Input: part model. Units: mm. Frame: model coordinates. Give positions to 0.01 mm unless a question says otherwise; leave off trailing zeros. Loops run counter-clockwise (first coordinate to the right, second up) from the corner with the lowest first, then second, coordinate; pieces in that order, holes last.
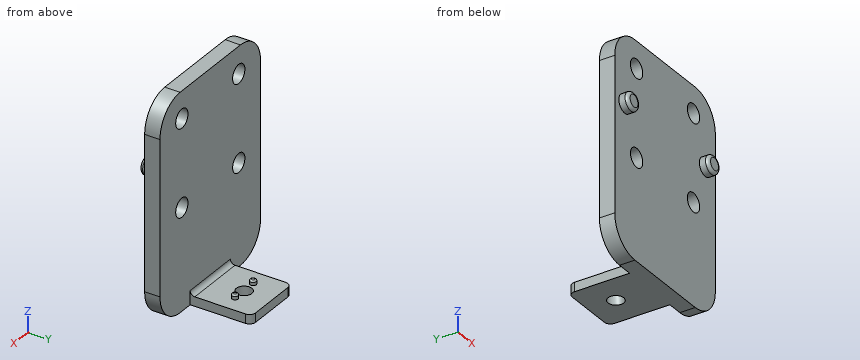
from build123d import *

# Parameters (mm, degrees)
SKETCH_1_W          = 50
SKETCH_1_H          = 70
EXTRUDE_1_DEPTH     = 5
SKETCH_2_R          = 3.05
CUT_EXTRUDE_1_DEPTH = 54.53308254
SKETCH_4_R          = 2.95
EXTRUDE_2_DEPTH     = 3
FILLET_1_R          = 1
FILLET_2_R          = 10
SKETCH_6_W          = 20
SKETCH_6_H          = 3
EXTRUDE_3_DEPTH     = 20
EXTRUDE_5_DEPTH     = 20
FILLET_3_R          = 2
SKETCH_9_R          = 2.55
CUT_EXTRUDE_2_DEPTH = 76.756187866
EXTRUDE_START       = 1.5
SKETCH_9_4_R        = 1
SKETCH_9_4_R_2      = 2.55
EXTRUDE_6_DEPTH     = 1.5
FILLET_4_R          = 0.5


with BuildPart() as part:
    # Sketch 1 → Extrude 1 (new body)
    with BuildSketch(Plane(origin=(0, 0, 0), x_dir=(1, 0, 0), z_dir=(0, 1, 0))):
        with Locations((0, 12.072188459)):
            Rectangle(SKETCH_1_W, SKETCH_1_H)
    extrude(amount=EXTRUDE_1_DEPTH)

    # Sketch 2 → Cut-Extrude 1 (cut, through all)
    with BuildSketch(Plane(origin=(0, 5, 0), x_dir=(1, 0, 0), z_dir=(0, 1, 0))):
        with Locations(Location((14.142135624, 14.142135624, 0), (0, 0, 270))):
            Circle(SKETCH_2_R)
        with Locations(Location((14.142135624, -14.142135624, 0), (0, 0, 270))):
            Circle(SKETCH_2_R)
        with Locations(Location((-14.142135624, -14.142135624, 0), (0, 0, 270))):
            Circle(SKETCH_2_R)
        with Locations(Location((-14.142135624, 14.142135624, 0), (0, 0, 270))):
            Circle(SKETCH_2_R)
    extrude(amount=-CUT_EXTRUDE_1_DEPTH, mode=Mode.SUBTRACT)

    # Sketch 4 → Extrude 2 (add)
    with BuildSketch(Plane.XZ):
        with Locations(Location((20, 0, 0), (0, 0, 90))):
            Circle(SKETCH_4_R)
        with Locations(Location((-20, 0, 0), (0, 0, 90))):
            Circle(SKETCH_4_R)
    extrude(amount=EXTRUDE_2_DEPTH)

    # Fillet 1
    fillet_1_edges = [part.edges().sort_by_distance(p)[0] for p in [
        (20, -3, -2.95),
        (-20, -3, -2.95),
    ]]
    fillet(fillet_1_edges, radius=FILLET_1_R)

    # Fillet 2
    fillet_2_edges = [part.edges().sort_by_distance(p)[0] for p in [
        (-25, 2.5, -47.072188459),
        (25, 2.5, -47.072188459),
        (25, 2.5, 22.927811541),
        (-25, 2.5, 22.927811541),
    ]]
    fillet(fillet_2_edges, radius=FILLET_2_R)

    # Sketch 6 → Extrude 3 (add)
    with BuildSketch(Plane(origin=(0, 5, 0), x_dir=(1, 0, 0), z_dir=(0, 1, 0))):
        with Locations((0, 45.572188459)):
            Rectangle(SKETCH_6_W, SKETCH_6_H)
    extrude(amount=EXTRUDE_3_DEPTH)

    # Sketch 8 → Extrude 5 (add)
    with BuildSketch(Plane.ZY.offset(10)):
        with BuildLine():
            Line((-44.072188459, 6.5), (-44.072188459, 5))
            Line((-44.072188459, 5), (-42.572188459, 5))
            ThreePointArc((-42.572188459, 5), (-43.63284863, 5.439339828), (-44.072188459, 6.5))
        make_face()
    extrude(amount=-EXTRUDE_5_DEPTH)

    # Fillet 3
    fillet_3_edges = [part.edges().sort_by_distance(p)[0] for p in [
        (-10, 25, -45.572188459),
        (10, 25, -45.572188459),
    ]]
    fillet(fillet_3_edges, radius=FILLET_3_R)

    # Sketch 9 → Cut-Extrude 2 (cut, through all)
    with BuildSketch(Plane.XY.offset(-44.072188459)):
        with Locations((0, 16)):
            Circle(SKETCH_9_R)
    extrude(amount=-CUT_EXTRUDE_2_DEPTH, mode=Mode.SUBTRACT)

    # Sketch 9_4 → Extrude 6 (add)
    with BuildSketch(Plane.XY.offset(-44.072188459).offset(EXTRUDE_START)):
        with Locations(Location((-4.5, 16, 0), (0, 0, 180))):
            Circle(SKETCH_9_4_R)
        with Locations(Location((4.5, 16, 0), (0, 0, 180))):
            Circle(SKETCH_9_4_R)
        with Locations((0, 16)):
            Circle(SKETCH_9_4_R_2)
    extrude(amount=-EXTRUDE_6_DEPTH)


with BuildPart() as extrude_6_kept_piece:
    # of the separate pieces the step leaves, the one the design keeps (extrude_6_pieces_kept)
    add(part.part.solids().sort_by_distance((10, 23, -47.072188459))[0])

    # Fillet 4
    fillet_4_edges = [extrude_6_kept_piece.edges().sort_by_distance(p)[0] for p in [
        (-3.5, 16, -42.572188459),
        (5.5, 16, -42.572188459),
    ]]
    fillet(fillet_4_edges, radius=FILLET_4_R)


solid = extrude_6_kept_piece.part
(1) Cut plane A-A (z = -15). Return the cut outline in (x, y), and give its area (3 significant figures).
Values follow:
outline: (-25, 0) - (-17.07, 0) - (-17.07, 5) - (-25, 5) - close; (-11.22, 0) - (11.22, 0) - (11.22, 5) - (-11.22, 5) - close; (17.07, 0) - (25, 0) - (25, 5) - (17.07, 5) - close
area: 191 mm2
(2) Cut plane C-C (y = 2.5). Return the cut outline in (x, z).
Values follow:
outline: (-25, -37.07) arc R10 ccw to (-15, -47.07) - (15, -47.07) arc R10 ccw to (25, -37.07) - (25, 12.93) arc R10 ccw to (15, 22.93) - (-15, 22.93) arc R10 ccw to (-25, 12.93) - close; hole circle Ø6.1 at (-14.14, -14.14); hole circle Ø6.1 at (-14.14, 14.14); hole circle Ø6.1 at (14.14, -14.14); hole circle Ø6.1 at (14.14, 14.14)
(3) Pin query (flat end, axial travel): pin 1 Ø0.5 at (x, y) = (-4.5, 16) entering from +Z; pin 2 Ø5 at (y, z) = (14.5, -44.5) entering from -X; pin 3 Ø8 at (y, z) = (15.5, -39) entering from +X. Return the tip coordinate at first contact, or that it passes through.
Values follow:
pin 1: stops at z = -42.57
pin 2: stops at x = -10
pin 3: stops at x = 5.49
(4) Cut plane B-B (x = -16). Return the cut outline in (y, z), and give its area (3 significant figures).
Values follow:
outline: (0, -47.02) - (5, -47.02) - (5, -16.56) - (0, -16.56) - close; (0, -11.72) - (5, -11.72) - (5, 11.72) - (0, 11.72) - close; (0, 16.56) - (5, 16.56) - (5, 22.88) - (0, 22.88) - close
area: 301 mm2
(5) Ray query, probe 1 along Y at (x, z) = (0, -45.6); probe 2 along X at (y, z) = (2.75, -11.5); probe 3 along Y at (x, z) = (-8, -23). Return the intervals inside material, ascending.
Values follow:
probe 1: y = 0 to 13.45, 18.55 to 25
probe 2: x = -25 to -15.67, -12.62 to 12.62, 15.67 to 25
probe 3: y = 0 to 5
(6) Cut plane D-D (z = 0). Return the cut outline in (x, y).
Values follow:
outline: (-25, 0) - (-22.95, 0) - (-22.95, -2) arc R1 ccw to (-21.95, -3) - (-18.05, -3) arc R1 ccw to (-17.05, -2) - (-17.05, 0) - (17.05, 0) - (17.05, -2) arc R1 ccw to (18.05, -3) - (21.95, -3) arc R1 ccw to (22.95, -2) - (22.95, 0) - (25, 0) - (25, 5) - (-25, 5) - close
